from build123d import *

# Parameters (mm, degrees)
SKETCH1_W           = 65.5
SKETCH1_H           = 30.5
BOSS_EXTRUDE1_DEPTH = 0.8
FILLET1_R           = 3.75
SKETCH2_R           = 1.375
CUT_EXTRUDE1_DEPTH  = 0.8
SKETCH3_W           = 30
SKETCH3_H           = 2.54
SKETCH3_W_2         = 9.253232542
SKETCH3_H_2         = 7.5
SKETCH3_W_3         = 15.108584743
SKETCH3_W_4         = 2.54
SKETCH3_W_5         = 15.573110358
SKETCH3_H_3         = 7.975960023
SKETCH3_W_6         = 5
SKETCH3_W_7         = 7.975960023
SKETCH3_H_4         = 7.78655518
BOSS_EXTRUDE2_DEPTH = 8
SKETCH4_W           = 51
SKETCH4_H           = 4.95
BOSS_EXTRUDE3_DEPTH = 4


with BuildPart() as part:
    # Sketch1 → Boss-Extrude1 (new body)
    with BuildSketch(Plane(origin=(0, 0, 0), x_dir=(1, 0, 0), z_dir=(0, 1, 0))):
        Rectangle(SKETCH1_W, SKETCH1_H)
    extrude(amount=BOSS_EXTRUDE1_DEPTH)

    # Fillet1
    fillet1_edges = [part.edges().sort_by_distance(p)[0] for p in [
        (-32.75, 0.4, -15.25),
        (32.75, 0.4, -15.25),
        (32.75, 0.4, 15.25),
        (-32.75, 0.4, 15.25),
    ]]
    fillet(fillet1_edges, radius=FILLET1_R)

    # Sketch2 → Cut-Extrude1 (cut)
    with BuildSketch(Plane(origin=(0, 0.8, 0), x_dir=(1, 0, 0), z_dir=(0, 1, 0))):
        with Locations(Location((-29, 11.5, 0), (0, 0, 270))):
            Circle(SKETCH2_R)
        with Locations(Location((-29, -11.5, 0), (0, 0, 270))):
            Circle(SKETCH2_R)
        with Locations(Location((29, -11.5, 0), (0, 0, 270))):
            Circle(SKETCH2_R)
        with Locations(Location((29, 11.5, 0), (0, 0, 270))):
            Circle(SKETCH2_R)
    extrude(amount=-CUT_EXTRUDE1_DEPTH, mode=Mode.SUBTRACT)

    # Sketch3 → Boss-Extrude2 (add)
    with BuildSketch(Plane(origin=(0, 0.8, 0), x_dir=(1, 0, 0), z_dir=(0, 1, 0))):
        with Locations((-15.426255017, 5.90276931)):
            Rectangle(SKETCH3_W, SKETCH3_H)
        with Locations((-6.452192743, -0.859199982)):
            Rectangle(SKETCH3_W_2, SKETCH3_H_2)
        with Locations((-21.80689744, -0.859199982)):
            Rectangle(SKETCH3_W_3, SKETCH3_H_2)
        with Locations((0.91413656, -8.040321366)):
            Rectangle(SKETCH3_W_4, SKETCH3_H_2)
        with Locations((15.976005132, -10.794375696)):
            Rectangle(SKETCH3_W_5, SKETCH3_H_3)
        with Locations((22.955137287, 1.585350321)):
            Rectangle(SKETCH3_W_4, SKETCH3_H_2)
        with Locations((12.438021136, -5.10451856)):
            Rectangle(SKETCH3_W_6, SKETCH3_H)
        with Locations((19.513989128, -5.10451856)):
            Rectangle(SKETCH3_W_6, SKETCH3_H)
        with Locations((28.644994423, 1.585350321)):
            Rectangle(SKETCH3_W_7, SKETCH3_H_4)
    extrude(amount=BOSS_EXTRUDE2_DEPTH)

    # Sketch4 → Boss-Extrude3 (add)
    with BuildSketch(Plane.XZ):
        with Locations((-0.25, -11.275)):
            Rectangle(SKETCH4_W, SKETCH4_H)
    extrude(amount=BOSS_EXTRUDE3_DEPTH)


solid = part.part
Can you work these out from the model? Positions are in its coordinate system, mm. A direction names the side the tool comes from. Give positions to 0.01 mm unless a question says otherwise; leave off trailing zeros. Loops run counter-clockwise (first coordinate to the right, second up) from the corner with the lowest first, then second, coordinate; pieces in that order, holes last. Notation, with made-up numbers: (28, 32) - (72, 32) arc R35 ccw to (72, 65) - close; hole circle Ø1 at (73, 14.5). An arc over 180 degrees is marked (long way). Return JSON: item names as keys, results as strings.
1. I want a section at A-A on z = 5.5. Please give me the cut outline in (x, y).
Output values:
{"outline": "(-32.75, 0) - (32.75, 0) - (32.75, 0.8) - (22.01, 0.8) - (22.01, 8.8) - (17.01, 8.8) - (17.01, 0.8) - (14.94, 0.8) - (14.94, 8.8) - (9.94, 8.8) - (9.94, 0.8) - (2.18, 0.8) - (2.18, 8.8) - (-0.36, 8.8) - (-0.36, 0.8) - (-32.75, 0.8) - close"}
2. If I drill on line 1 (X direction, y = 0.6, z = -11.5) (3 decimals); line 2 (X direction, y = 1.25, z = -2); line 3 (X direction, y = 3.25, z = 5.5), over which ranges is the centre line in solid material (lowest first)?
Output values:
{"line 1": "x = -32.75 to -30.375, -27.625 to 27.625, 30.375 to 32.75", "line 2": "x = -29.36 to -14.25, -11.08 to -1.83, 21.69 to 24.23, 24.66 to 32.63", "line 3": "x = -0.36 to 2.18, 9.94 to 14.94, 17.01 to 22.01"}
3. I want a section at C-C on y = 3.25. Give the number of separate pieces and of enclosed holes in the cut face, and give its area (3 significant figures).
Output values:
{"separate pieces": "9", "enclosed holes": "0", "area": "509 mm²"}
4. I'm going to push flat-ended pins straight in: pin 1 Ø1.5 at (x, y) = (-10.5, 5) entering from +Z; pin 2 Ø3 at (x, z) = (29, 11.5) entering from +Y; pin 3 Ø3 at (x, y) = (23.5, 5.5) entering from +Z. Where does each tip first touch, or does it pass through?
Output values:
{"pin 1": "stops at z = 4.61", "pin 2": "stops at y = 0.8", "pin 3": "stops at z = 14.78"}
5. For faces 4 (the face through (-14.253, 5, 1)), 5 (the face through (-29.361, 5, 1)), 6 (the face through (1, 5, 4.29)), which set-ups out of +Z, -Z, +X, -X, +Y, -Y let a thin tool reach every point of the face, with its end or its side?
Output values:
{"face 4": "+Z, +Y", "face 5": "+Z, -X, +Y", "face 6": "-Z, +Y"}
6. We'd pull the mould along Z, two halves only. Please class faces 1 (the face through (19, 5, 6.375)), 2 (the face through (9.938, 5, 5)), 3 (the face through (23, 5, -5.335)): +Z half, -Z half, draft (parallel to the pull), parting line (faces both ways), or undercut.
Output values:
{"face 1": "undercut", "face 2": "draft", "face 3": "-Z half"}
7. I want a section at B-B on x = -23.5. Please give me the cut outline in (y, z).
Output values:
{"outline": "(-4, -13.75) - (0, -13.75) - (0, -15.25) - (0.8, -15.25) - (0.8, -7.17) - (8.8, -7.17) - (8.8, -4.63) - (0.8, -4.63) - (0.8, -2.89) - (8.8, -2.89) - (8.8, 4.61) - (0.8, 4.61) - (0.8, 15.25) - (0, 15.25) - (0, -8.8) - (-4, -8.8) - close"}
